from build123d import *

# Parameters (mm, degrees)
SKETCH1_W           = 110.936328641
SKETCH1_H           = 74.919128642
BOSS_EXTRUDE1_DEPTH = 3.175
SKETCH2_R           = 3.175
CUT_EXTRUDE1_DEPTH  = 4.175
SKETCH10_R          = 3.175
CUT_EXTRUDE5_DEPTH  = 4.175
CUT_EXTRUDE6_DEPTH  = 4.175
SKETCH12_R          = 3.370079304
SKETCH12_R_2        = 3.429
CUT_EXTRUDE7_DEPTH  = 4.175


with BuildPart() as part:
    # Sketch1 → Boss-Extrude1 (new body)
    with BuildSketch(Plane(origin=(0, 0, 0), x_dir=(1, 0, 0), z_dir=(0, 1, 0))):
        with Locations((-27.986559238, -0.898578046)):
            Rectangle(SKETCH1_W, SKETCH1_H)
    extrude(amount=BOSS_EXTRUDE1_DEPTH)

    # Sketch2 → Cut-Extrude1 (cut, through all)
    with BuildSketch(Plane.XZ):
        with Locations((-77.473379238, 32.394578046)):
            Circle(SKETCH2_R)
    extrude(amount=-CUT_EXTRUDE1_DEPTH, mode=Mode.SUBTRACT)

    # Sketch10 → Cut-Extrude5 (cut, through all)
    with BuildSketch(Plane(origin=(0, 3.175, 0), x_dir=(1, 0, 0), z_dir=(0, 1, 0))):
        with Locations((3.519600762, -23.395358046)):
            Circle(SKETCH10_R)
        with Locations((12.518820762, 12.601521954)):
            Circle(SKETCH10_R)
    extrude(amount=-CUT_EXTRUDE5_DEPTH, mode=Mode.SUBTRACT)

    # Sketch11 → Cut-Extrude6 (cut, through all)
    with BuildSketch(Plane(origin=(0, 3.175, 0), x_dir=(1, 0, 0), z_dir=(0, 1, 0))):
        with BuildLine():
            Line((-78.770441311, -16.175423663), (-78.770441311, 21.600741954))
            ThreePointArc((-78.770441311, 21.600741954), (-77.473379238, 22.897804027), (-76.176317164, 21.600741954))
            Line((-76.176317164, 21.600741954), (-76.176317164, -16.175423663))
            ThreePointArc((-76.176317164, -16.175423663), (-77.473379238, -17.472485737), (-78.770441311, -16.175423663))
        make_face()
        with BuildLine():
            Line((-59.474939238, 31.899342378), (12.518820762, 31.899342378))
            ThreePointArc((12.518820762, 31.899342378), (13.818201186, 30.599961954), (12.518820762, 29.30058153))
            Line((12.518820762, 29.30058153), (-59.474939238, 29.30058153))
            ThreePointArc((-59.474939238, 29.30058153), (-60.774319661, 30.599961954), (-59.474939238, 31.899342378))
        make_face()
        with BuildLine():
            Line((12.518820762, -33.852545554), (-59.474939238, -33.852545554))
            ThreePointArc((-59.474939238, -33.852545554), (-60.932906745, -32.394578046), (-59.474939238, -30.936610538))
            Line((-59.474939238, -30.936610538), (12.518820762, -30.936610538))
            ThreePointArc((12.518820762, -30.936610538), (13.97678827, -32.394578046), (12.518820762, -33.852545554))
        make_face()
        with BuildLine():
            Line((20.226413943, -16.175423663), (20.226413943, 21.600741954))
            ThreePointArc((20.226413943, 21.600741954), (21.518040762, 22.892368774), (22.809667582, 21.600741954))
            Line((22.809667582, 21.600741954), (22.809667582, -16.175423663))
            ThreePointArc((22.809667582, -16.175423663), (21.518040762, -17.467050483), (20.226413943, -16.175423663))
        make_face()
    extrude(amount=-CUT_EXTRUDE6_DEPTH, mode=Mode.SUBTRACT)

    # Sketch12 → Cut-Extrude7 (cut, through all)
    with BuildSketch(Plane(origin=(0, 3.175, 0), x_dir=(1, 0, 0), z_dir=(0, 1, 0))):
        with Locations((-68.474159238, 21.600741954)):
            Circle(SKETCH12_R)
        with Locations((-32.477279238, -5.396918046)):
            Circle(SKETCH12_R_2)
        with Locations((-5.479619238, 12.601521954)):
            Circle(SKETCH12_R_2)
    extrude(amount=-CUT_EXTRUDE7_DEPTH, mode=Mode.SUBTRACT)


solid = part.part
Verification items for the finished model (mm, model axes). A direction names the side the tool comes from. Give positions to 0.01 mm unless a question says otherwise; leave off trailing zeros. Write each loop counter-clockwise with the first axis right and the second up, starting at its lowest first coordinate (ties: lowest second). Pieces come first, ordered by that corner, then holes. Notation, with made-up numbers: M 35.5,-16 L 64.5,-16 A37 ccw 64.5,20 Z; hole C -28.5,77.5 d11. An arc over 180 degrees is marked long. Write item = value, one per line.
(1) Sectioned sample at D-D (x = -7). Record the cut outline in (y, z) (3 decimals), then the cut area to 3 significant figures.
Found:
outline = M 0,-36.561 L 3.175,-36.561 L 3.175,-31.899 L 0,-31.899 Z; M 0,-29.301 L 3.175,-29.301 L 3.175,-15.675 L 0,-15.675 Z; M 0,-9.528 L 3.175,-9.528 L 3.175,30.937 L 0,30.937 Z; M 0,33.853 L 3.175,33.853 L 3.175,38.358 L 0,38.358 Z
area = 201 mm2
(2) Sectioned sample at A-A (z = 15). Record the cut outline in (x, y) (3 decimals).
Found:
outline = M -83.455,0 L -78.77,0 L -78.77,3.175 L -83.455,3.175 Z; M -76.176,0 L 20.226,0 L 20.226,3.175 L -76.176,3.175 Z; M 22.81,0 L 27.482,0 L 27.482,3.175 L 22.81,3.175 Z
(3) Access from +Z, -Z, +X, -X, +Y, -Y to the whole of each face (thin tool, end or side, straight path). Record for faces 1 (the face through (-23, 2, 33.853)), 2 (the face through (-29, 2, 38.358)).
Found:
face_1 = +Y, -Y
face_2 = +Z, +X, -X, +Y, -Y
(4) Material ranges on line 1 (Z direction, x = -10, y = 2.65); line 2 (X direction, y = 0.5, z = 1.5); line 3 (Z direction, x = -32.5, y = 2.45), recorded low to high.
Found:
line_1 = -36.56 to -31.9, -29.3 to 30.94, 33.85 to 38.36
line_2 = -83.45 to -78.77, -76.18 to 20.23, 22.81 to 27.48
line_3 = -36.56 to -31.9, -29.3 to 1.97, 8.83 to 30.94, 33.85 to 38.36
(5) Sectioned sample at B-B (x = -49). Record the cut outline in (y, z) (3 decimals), then the cut area to 3 significant figures.
Found:
outline = M 0,-36.561 L 3.175,-36.561 L 3.175,-31.899 L 0,-31.899 Z; M 0,-29.301 L 3.175,-29.301 L 3.175,30.937 L 0,30.937 Z; M 0,33.853 L 3.175,33.853 L 3.175,38.358 L 0,38.358 Z
area = 220 mm2
(6) Sectioned sample at C-C (z = -11). Record the cut outline in (x, y) (3 decimals), then the cut area to 3 significant figures.
Found:
outline = M -83.455,0 L -78.77,0 L -78.77,3.175 L -83.455,3.175 Z; M -76.176,0 L -8.512,0 L -8.512,3.175 L -76.176,3.175 Z; M -2.448,0 L 9.777,0 L 9.777,3.175 L -2.448,3.175 Z; M 15.26,0 L 20.226,0 L 20.226,3.175 L 15.26,3.175 Z; M 22.81,0 L 27.482,0 L 27.482,3.175 L 22.81,3.175 Z
area = 299 mm2
